Design review of the part built by this model. Coordinates are the model's own, in mm. A direction names the side the tool comes from. Round coordinates to 2 decimals unless told otherwise and drop trailing zeros. Loops run counter-clockwise (first coordinate to the right, second up) from the corner with the lowest first, then second, coordinate; pieces in that order, holes last. Notation, with made-up numbers: (60.25, 70) -> (119.25, 70) arc R15 ccw to (119.25, 85) -> close; hole circle Ø7 at (48, 30.5). An arc over 180 degrees is marked (long way). Write each question's results on one line, items separated by ' | '. Start each with the question number.
from build123d import *

# Parameters (mm, degrees)
BOSS_EXTRUDE2_DEPTH                                 = 20
SKETCH3_R                                           = 18.625
CUT_EXTRUDE1_DEPTH                                  = 18
SKETCH5_R                                           = 7.5
CUT_EXTRUDE2_DEPTH                                  = 2
CSK_FOR_M3_COUNTERSUNK_FLAT_HEAD_SCREW2_D           = 3.5
CSK_FOR_M3_COUNTERSUNK_FLAT_HEAD_SCREW2_CSINK_D     = 5.5
CSK_FOR_M3_COUNTERSUNK_FLAT_HEAD_SCREW2_CSINK_ANGLE = 90


with BuildPart() as part:
    # Sketch1 → Boss-Extrude2 (new body)
    with BuildSketch(Plane(origin=(0, 0, 0), x_dir=(1, 0, 0), z_dir=(0, 1, 0))):
        with BuildLine():
            Line((-18.727852322, -5.86584797), (-18.727852322, -15.86584797))
            Line((-18.727852322, -15.86584797), (-30.687012052, -15.86584797))
            Line((-30.687012052, -15.86584797), (-30.687012052, -18.86584797))
            Line((-30.687012052, -18.86584797), (-15.687012052, -18.86584797))
            Line((-15.687012052, -18.86584797), (-15.687012052, -11.792297397))
            Line((-15.687012052, -11.792297397), (15.687012052, -11.366724546))
            Line((15.687012052, -11.366724546), (15.687012052, -18.86584797))
            Line((15.687012052, -18.86584797), (30.687012052, -18.86584797))
            Line((30.687012052, -18.86584797), (30.687012052, -15.86584797))
            Line((30.687012052, -15.86584797), (18.727852322, -15.86584797))
            Line((18.727852322, -15.86584797), (18.727852322, -5.86584797))
            ThreePointArc((18.727852322, -5.86584797), (0, 19.625), (-18.727852322, -5.86584797))
        make_face()
    extrude(amount=BOSS_EXTRUDE2_DEPTH)

    # Sketch3 → Cut-Extrude1 (cut)
    with BuildSketch(Plane(origin=(0, 20, 0), x_dir=(1, 0, 0), z_dir=(0, 1, 0))):
        Circle(SKETCH3_R)
    extrude(amount=-CUT_EXTRUDE1_DEPTH, mode=Mode.SUBTRACT)

    # Sketch5 → Cut-Extrude2 (cut)
    with BuildSketch(Plane(origin=(0, 2, 0), x_dir=(1, 0, 0), z_dir=(0, 1, 0))):
        with Locations((-0.094951478, -7)):
            Circle(SKETCH5_R)
    extrude(amount=-CUT_EXTRUDE2_DEPTH, mode=Mode.SUBTRACT)

    # CSK for M3 Countersunk Flat Head Screw2 (through all)
    with Locations(Plane(origin=(7.75, 0, -13.423393759), x_dir=(0, 0, -1), z_dir=(0, -1, 0))):
        with Locations((0, 0), (0, -15.5), (-13.423393759, -23.25), (-13.423393759, 7.75)):
            CounterSinkHole(CSK_FOR_M3_COUNTERSUNK_FLAT_HEAD_SCREW2_D / 2, CSK_FOR_M3_COUNTERSUNK_FLAT_HEAD_SCREW2_CSINK_D / 2, counter_sink_angle=CSK_FOR_M3_COUNTERSUNK_FLAT_HEAD_SCREW2_CSINK_ANGLE)


solid = part.part
1) Take a section at C-C (z = -14). State how many separate pieces and enclosed holes the cut face has, plus the area to 3 significant figures.
2) The part is to be moulded in two halves that separate along X. For faces 1 (the face through (0, 1, -0.5)), 2 (the face through (25, 10, 15.866)), 3 (the face through (-30.687, 10, 17)), 4 (the face through (15.687, 10, 15)), say which applies: +X half, -X half, draft (parallel to the pull), parting line (faces both ways), or undercut.
3) Insertion check: pin 1 (8 mm diameter, centred on x = 9.5, y = 10.5, fed in from +Z); pin 2 (3 mm diameter, centred on y = 11, z = -14.5, fed in from +X); pin 3 (4 mm diameter, centred on y = 12.5, z = 4.5, fed in from +X). Each pin has a flat end and moves straight along its axis. Give the tip position at first contact, or say it passes through.
4) To check wall thickness, follow line 1 (X direction, y = 11.75, z = 12.5); line 2 (Y direction, x = 5, z = -9); line 3 (Z direction, x = -22.5, y = 7.75). State the ranges of each line that lie inside material, in increasing order. Write a range as from..to.
5) For faces 5 (the face through (0, 2, -4)), 6 (the face through (-15.687, 10, 15)), 7 (the face through (-16, 20, 10)), list the 3-axis set-ups (+Z, -Z, +X, -X, +Y, -Y) from which the entire face can be reached by the end or side of a thin tool; tool diameter is ignored.
6) Take a section at B-B (z = -6.5). Write out the cut boundary in (x, y).
7) Take a section at A-A (y = 14.25). Write out the cut boundary in (x, z) (3 decimals).
8) Take a section at D-D (x = 0). Write out the cut boundary in (y, z) (3 decimals), plus the area to 3 significant figures.
Geometry check:
1) separate pieces: 3 | enclosed holes: 0 | area: 92.6 mm^2
2) face 1: undercut | face 2: draft | face 3: -X half | face 4: undercut
3) pin 1: stops at z = -12.83 | pin 2: stops at x = 14.7 | pin 3: stops at x = 19.47
4) line 1: x = -18.73..-15.69, 15.69..18.73 | line 2: y = 0..2 | line 3: z = 15.87..18.87
5) face 5: +Y | face 6: +Z, +Y, -Y | face 7: +Z, -Z, +X, -X, +Y
6) outline: (-18.52, 0) -> (18.52, 0) -> (18.52, 20) -> (17.45, 20) -> (17.45, 2) -> (-17.45, 2) -> (-17.45, 20) -> (-18.52, 20) -> close
7) outline: (-30.687, 15.866) -> (-18.728, 15.866) -> (-18.728, 5.866) arc R19.625 ccw (long way) to (18.728, 5.866) -> (18.728, 15.866) -> (30.687, 15.866) -> (30.687, 18.866) -> (15.687, 18.866) -> (15.687, 11.367) -> (14.744, 11.38) arc R18.625 cw (long way) to (-14.43, 11.775) -> (-15.687, 11.792) -> (-15.687, 18.866) -> (-30.687, 18.866) -> close
8) outline: (0, -19.625) -> (20, -19.625) -> (20, -18.625) -> (2, -18.625) -> (2, -0.499) -> (0, -0.499) -> close | area: 56.3 mm^2
